Can you work these out from the model? Positions are in its coordinate system, mm. A direction names the side the tool comes from. Round coordinates to 2 decimals unless told otherwise and drop trailing zeros. Write each loop counter-clockwise with the first axis right and the second up, starting at its lowest first coordinate (ties: lowest second). Pieces come first, ordered by that corner, then holes.
Q1. If we section it at D-D (z = -43): Please give me the cut outline in (x, y).
Q2. Please list where these lines run through material, in increasing order: line 1 along X through (y, z) = (2.9, -53); line 2 along Y through (x, z) = (44, -30.5); line 3 along Z through (x, y) = (5.5, 2.9).
Q3. If we section it at C-C (z = -49.5): Please give me the cut outline in (x, y), plus the area to 3 significant figures.
Q4. We'd pull the mould along Z, two halves only. Please class faces 1 (the flat face through (4, 5.5, -56)), 2 (the flat face through (78, 3, -48.38)), 3 (the flat face through (6, 3, -57.38)): +Z half, -Z half, draft (parallel to the pull), parting line (faces both ways), or undercut.
Q5. For faces 4 (the flat face through (74, 3, -57.38)), 5 (the flat face through (2, 3, -10.51)), 6 (the flat face through (3.51, 3, -52)), 7 (the flat face through (78.49, 3, -7)), which set-ups out of +Z, -Z, +X, -X, +Y, -Y let a thin tool reach every point of the face, with its end or its side?
Q6. I'm going to push flat-ended pins straight in: pin 1 Ø6 at (x, z) = (24, -21.5) entering from -Y; pin 2 Ø2 at (x, y) = (77, 4) entering from +Z; pin 3 Ø2 at (x, y) = (3, 4) entering from -Z; pin 4 Ø3 at (y, z) = (3.5, -54) entering from +X. Where does each tip first touch, or does it pass through?
Q7. If we section it at B-B (x = 6): Please give me the cut outline in (y, z), plus the area to 3 significant figures.
Q8. If we section it at A-A (y = 2.75): Please give me the cut outline in (x, z), plus the area to 3 significant figures.
Autodesk Fusion 360 part; units mm, degrees
sketch "Sketch1" plane through (0, 0, 0) normal (0, 1, 0) x (1, 0, 0)
  line L0 (0, 0) -> (80, 0)
  line L1 (80, 0) -> (80, 58.89)
  line L2 (80, 58.89) -> (0, 58.89)
  line L3 (0, 58.89) -> (0, 0)
  line L4 (46, 0) -> (34, 0)
  line L5 (34, 0) -> (34, 8)
  line L6 (34, 8) -> (46, 8)
  line L7 (46, 8) -> (46, 0)
  dimension "d1" = 58.89
  dimension "d2" = 80
  dimension "d11" = 8
  dimension "d14" = 12
  dimension "d15" = 34
extrude "Extrude1" add sketch "Sketch1" along normal blind 1.5
sketch "Sketch2" plane through (0, 1.5, 0) normal (0, 1, 0) x (-1, 0, 0)
  line L0 (0, -58.89) -> (0, 0)
  line L1 (0, 0) -> (-80, 0)
  line L2 (-80, 0) -> (-80, -58.89)
  line L3 (-80, -58.89) -> (0, -58.89)
  line L4 (-10.51, -1.51) -> (-1.51, -1.51)
  line L5 (-1.51, -1.51) -> (-1.51, -10.51)
  line L6 (-1.51, -10.51) -> (-10.51, -10.51)
  line L7 (-10.51, -10.51) -> (-10.51, -1.51)
  line L8 (-10.51, -10.51) -> (-3.51, -10.51)
  line L9 (-3.51, -10.51) -> (-3.51, -3.51)
  line L10 (-3.51, -3.51) -> (-10.51, -3.51)
  line L11 (-10.51, -3.51) -> (-10.51, -10.51)
  line L12 (0, -29.445) -> (-80, -29.445) construction
  line L13 (-3.51, -48.38) -> (-3.51, -55.38)
  line L14 (-3.51, -55.38) -> (-10.51, -55.38)
  line L15 (-10.51, -48.38) -> (-10.51, -57.38)
  line L16 (-1.51, -48.38) -> (-10.51, -48.38)
  line L17 (-1.51, -57.38) -> (-1.51, -48.38)
  line L18 (-10.51, -57.38) -> (-1.51, -57.38)
  line L19 (-69.49, -1.51) -> (-78.49, -1.51)
  line L20 (-76.49, -3.51) -> (-69.49, -3.51)
  line L21 (-78.49, -1.51) -> (-78.49, -10.51)
  line L22 (-76.49, -10.51) -> (-76.49, -3.51)
  line L23 (-78.49, -10.51) -> (-69.49, -10.51)
  line L24 (-69.49, -10.51) -> (-69.49, -1.51)
  line L25 (-78.49, -48.38) -> (-69.49, -48.38)
  line L26 (-69.49, -48.38) -> (-69.49, -57.38)
  line L27 (-76.49, -48.38) -> (-76.49, -55.38)
  line L28 (-78.49, -57.38) -> (-78.49, -48.38)
  line L29 (-76.49, -55.38) -> (-69.49, -55.38)
  line L30 (-69.49, -57.38) -> (-78.49, -57.38)
  line L31 (-3.51, -3.51) -> (-1.51, -3.51)
  line L32 (-76.49, -3.51) -> (-78.49, -3.51)
  dimension "d5" = 9
  dimension "d6" = 9
  dimension "d7" = 1.51
  dimension "d8" = 1.51
extrude "Extrude2" add sketch "Sketch2" along normal blind 4 contours L5 L6 L9 L31 | L13 L14 L15 L16 L17 L18 | L21 L22 L23 L32 | L25 L26 L27 L28 L29 L30
extrude "Extrude3" cut sketch "Sketch1" against normal blind 8.263 contours L0 L4 L5 L6 L7
A:
1. outline: (0, 0) - (80, 0) - (80, 1.5) - (0, 1.5) - close
2. line 1: x = 1.51 to 3.51, 76.49 to 78.49
2. line 2: y = 0 to 1.5
2. line 3: z = -57.38 to -55.38
3. outline: (0, 0) - (80, 0) - (80, 1.5) - (78.49, 1.5) - (78.49, 5.5) - (76.49, 5.5) - (76.49, 1.5) - (3.51, 1.5) - (3.51, 5.5) - (1.51, 5.5) - (1.51, 1.5) - (0, 1.5) - close
3. area: 136 mm2
4. face 1: draft
4. face 2: undercut
4. face 3: -Z half
5. face 4: -Z, +X, -X, +Y
5. face 5: +X, -X, +Y
5. face 6: +Z, +Y
5. face 7: +Z, -Z, +X, +Y
6. pin 1: stops at y = 0
6. pin 2: stops at z = -3.51
6. pin 3: stops at z = -57.38
6. pin 4: stops at x = 78.49
7. outline: (0, -58.89) - (1.5, -58.89) - (1.5, -57.38) - (5.5, -57.38) - (5.5, -55.38) - (1.5, -55.38) - (1.5, 0) - (0, 0) - close
7. area: 96.3 mm2
8. outline: (1.51, -57.38) - (10.51, -57.38) - (10.51, -55.38) - (3.51, -55.38) - (3.51, -48.38) - (1.51, -48.38) - close; (1.51, -10.51) - (3.51, -10.51) - (3.51, -3.51) - (1.51, -3.51) - close; (69.49, -57.38) - (78.49, -57.38) - (78.49, -48.38) - (76.49, -48.38) - (76.49, -55.38) - (69.49, -55.38) - close; (76.49, -10.51) - (78.49, -10.51) - (78.49, -3.51) - (76.49, -3.51) - close
8. area: 92.0 mm2
